Can you work these out from the model? Positions are in its coordinate system, mm. Face numbers are marked on the shaded views. A direction names the side the tool comes from. Give positions to 0.01 mm unless a question says otherwise; leave off trailing zeros. Order: outer loops, then holes, each group sorted by start corner. A loop starts at its lowest first (then second) coordinate and runs counter-clockwise, first axis right, second up. Notation, with made-up numbers: (44.5, 62.25) -> (62.5, 62.25) arc R31 ccw to (62.5, 92.25) -> close; hole circle Ø10 at (40.25, -30). An arc over 180 degrees is marked (long way). Answer as CSV lines item,"result".
```python
from build123d import *

# Parameters (mm, degrees)
SKETCH2_OUTSIDE_W                   = 55.422
SKETCH2_OUTSIDE_H                   = 55.422
CUT_EXTRUDE_PUSHER_SIDE_CROSS_DEPTH = 103.124
CUT_EXTRUDE_CROSS_2_DEPTH           = 3.048
SKETCH8_OUTSIDE_W                   = 55.422
SKETCH8_OUTSIDE_H                   = 55.422
CUT_EXTRUDE1_DEPTH                  = 3.54


with BuildPart() as part:
    # Sketch1 → Revolve: Main Body (revolve)
    with BuildSketch(Plane.XY):
        with BuildLine():
            Line((0, 0), (0, 14.605))
            Line((0, 14.605), (1.651, 14.605))
            Line((1.651, 14.605), (1.651, 11.7348))
            Line((1.651, 11.7348), (106.68, 11.7348))
            Line((106.68, 11.7348), (106.68, 9.5885))
            Line((106.68, 9.5885), (111.252, 9.5885))
            Line((111.252, 9.5885), (111.252, 8.89))
            Line((111.252, 8.89), (113.775706947, 1.318879159))
            ThreePointArc((113.775706947, 1.318879159), (113.787900268, 1.269334705), (113.792, 1.218476843))
            Line((113.792, 1.218476843), (113.792, 0))
            Line((113.792, 0), (0, 0))
        make_face()
    revolve(axis=Axis((-3.305576832, 0, 0), (1, 0, 0)))

    # Sketch2 outside → Cut-Extrude: Pusher Side Cross (cut)
    with BuildSketch(Plane(origin=(1.651, 0, 0), x_dir=(0, 0, -1), z_dir=(1, 0, 0))):
        Rectangle(SKETCH2_OUTSIDE_W, SKETCH2_OUTSIDE_H)
        Polygon((-0.6985, 11.303), (0.6985, 11.303), (0.6985, 0.6985), (11.303, 0.6985), (11.303, -0.6985), (0.6985, -0.6985), (0.6985, -11.303), (-0.6985, -11.303), (-0.6985, -0.6985), (-11.303, -0.6985), (-11.303, 0.6985), (-0.6985, 0.6985), align=None, mode=Mode.SUBTRACT)
    extrude(amount=CUT_EXTRUDE_PUSHER_SIDE_CROSS_DEPTH, mode=Mode.SUBTRACT)

    # Sketch3 → Cut-Extrude: Cross 2 (cut)
    with BuildSketch(Plane(origin=(106.68, 0, 0), x_dir=(0, 0, -1), z_dir=(1, 0, 0))):
        with BuildLine():
            Line((-11.713992863, 0.6985), (-9.563024103, 0.6985))
            ThreePointArc((-9.563024103, 0.6985), (-6.780093371, 6.780093371), (-0.6985, 9.563024103))
            Line((-0.6985, 9.563024103), (-0.6985, 11.713992863))
            ThreePointArc((-0.6985, 11.713992863), (-8.297756656, 8.297756656), (-11.713992863, 0.6985))
        make_face()
        with BuildLine():
            Line((0.6985, 11.713992863), (0.6985, 9.563024103))
            ThreePointArc((0.6985, 9.563024103), (6.780093371, 6.780093371), (9.563024103, 0.6985))
            Line((9.563024103, 0.6985), (11.713992863, 0.6985))
            ThreePointArc((11.713992863, 0.6985), (8.297756656, 8.297756656), (0.6985, 11.713992863))
        make_face()
        with BuildLine():
            ThreePointArc((9.563024103, -0.6985), (6.780093371, -6.780093371), (0.6985, -9.563024103))
            Line((0.6985, -9.563024103), (0.6985, -11.713992863))
            ThreePointArc((0.6985, -11.713992863), (8.297756656, -8.297756656), (11.713992863, -0.6985))
            Line((11.713992863, -0.6985), (9.563024103, -0.6985))
        make_face()
        with BuildLine():
            ThreePointArc((-0.6985, -9.563024103), (-6.780093371, -6.780093371), (-9.563024103, -0.6985))
            Line((-9.563024103, -0.6985), (-11.713992863, -0.6985))
            ThreePointArc((-11.713992863, -0.6985), (-8.297756656, -8.297756656), (-0.6985, -11.713992863))
            Line((-0.6985, -11.713992863), (-0.6985, -9.563024103))
        make_face()
        with BuildLine():
            Line((-9.563024103, 0.6985), (-7.58791788, 0.6985))
            Line((-7.58791788, 0.6985), (-0.6985, 0.6985))
            Line((-0.6985, 0.6985), (-0.6985, 7.58791788))
            Line((-0.6985, 7.58791788), (-0.6985, 9.563024103))
            ThreePointArc((-0.6985, 9.563024103), (-6.780093371, 6.780093371), (-9.563024103, 0.6985))
        make_face()
        with BuildLine():
            Line((0.6985, 9.563024103), (0.6985, 7.58791788))
            Line((0.6985, 7.58791788), (0.6985, 0.6985))
            Line((0.6985, 0.6985), (7.58791788, 0.6985))
            Line((7.58791788, 0.6985), (9.563024103, 0.6985))
            ThreePointArc((9.563024103, 0.6985), (6.780093371, 6.780093371), (0.6985, 9.563024103))
        make_face()
        with BuildLine():
            Line((0.6985, -7.58791788), (0.6985, -9.563024103))
            ThreePointArc((0.6985, -9.563024103), (6.780093371, -6.780093371), (9.563024103, -0.6985))
            Line((9.563024103, -0.6985), (7.58791788, -0.6985))
            Line((7.58791788, -0.6985), (0.6985, -0.6985))
            Line((0.6985, -0.6985), (0.6985, -7.58791788))
        make_face()
        with BuildLine():
            Line((-0.6985, -0.6985), (-7.58791788, -0.6985))
            Line((-7.58791788, -0.6985), (-9.563024103, -0.6985))
            ThreePointArc((-9.563024103, -0.6985), (-6.780093371, -6.780093371), (-0.6985, -9.563024103))
            Line((-0.6985, -9.563024103), (-0.6985, -7.58791788))
            Line((-0.6985, -7.58791788), (-0.6985, -0.6985))
        make_face()
        with BuildLine():
            Line((-0.6985, -7.58791788), (-0.6985, -9.563024103))
            ThreePointArc((-0.6985, -9.563024103), (0, -9.5885), (0.6985, -9.563024103))
            Line((0.6985, -9.563024103), (0.6985, -7.58791788))
            ThreePointArc((0.6985, -7.58791788), (0, -7.62), (-0.6985, -7.58791788))
        make_face()
        with BuildLine():
            Line((-0.6985, 9.563024103), (-0.6985, 7.58791788))
            ThreePointArc((-0.6985, 7.58791788), (0, 7.62), (0.6985, 7.58791788))
            Line((0.6985, 7.58791788), (0.6985, 9.563024103))
            ThreePointArc((0.6985, 9.563024103), (0, 9.5885), (-0.6985, 9.563024103))
        make_face()
        with BuildLine():
            Line((-0.6985, 11.713992863), (-0.6985, 9.563024103))
            ThreePointArc((-0.6985, 9.563024103), (0, 9.5885), (0.6985, 9.563024103))
            Line((0.6985, 9.563024103), (0.6985, 11.713992863))
            ThreePointArc((0.6985, 11.713992863), (0, 11.7348), (-0.6985, 11.713992863))
        make_face()
        with BuildLine():
            ThreePointArc((0.6985, -9.563024103), (0, -9.5885), (-0.6985, -9.563024103))
            Line((-0.6985, -9.563024103), (-0.6985, -11.713992863))
            ThreePointArc((-0.6985, -11.713992863), (0, -11.7348), (0.6985, -11.713992863))
            Line((0.6985, -11.713992863), (0.6985, -9.563024103))
        make_face()
        with BuildLine():
            Line((11.713992863, 0.6985), (9.563024103, 0.6985))
            ThreePointArc((9.563024103, 0.6985), (9.582128909, 0.349482214), (9.5885, 0))
            ThreePointArc((9.5885, 0), (9.582128909, -0.349482214), (9.563024103, -0.6985))
            Line((9.563024103, -0.6985), (11.713992863, -0.6985))
            ThreePointArc((11.713992863, -0.6985), (11.729597062, -0.349404918), (11.7348, 0))
            ThreePointArc((11.7348, 0), (11.729597062, 0.349404918), (11.713992863, 0.6985))
        make_face()
        with BuildLine():
            ThreePointArc((9.5885, 0), (9.582128909, 0.349482214), (9.563024103, 0.6985))
            Line((9.563024103, 0.6985), (7.58791788, 0.6985))
            ThreePointArc((7.58791788, 0.6985), (7.62, 0), (7.58791788, -0.6985))
            Line((7.58791788, -0.6985), (9.563024103, -0.6985))
            ThreePointArc((9.563024103, -0.6985), (9.582128909, -0.349482214), (9.5885, 0))
        make_face()
        with BuildLine():
            ThreePointArc((-7.58791788, -0.6985), (-7.62, 0), (-7.58791788, 0.6985))
            Line((-7.58791788, 0.6985), (-9.563024103, 0.6985))
            ThreePointArc((-9.563024103, 0.6985), (-9.5885, 0), (-9.563024103, -0.6985))
            Line((-9.563024103, -0.6985), (-7.58791788, -0.6985))
        make_face()
        with BuildLine():
            ThreePointArc((-9.563024103, -0.6985), (-9.5885, 0), (-9.563024103, 0.6985))
            Line((-9.563024103, 0.6985), (-11.713992863, 0.6985))
            ThreePointArc((-11.713992863, 0.6985), (-11.7348, 0), (-11.713992863, -0.6985))
            Line((-11.713992863, -0.6985), (-9.563024103, -0.6985))
        make_face()
    extrude(amount=CUT_EXTRUDE_CROSS_2_DEPTH, mode=Mode.SUBTRACT)

    # Sketch8 outside → Cut-Extrude1 (cut, through all)
    with BuildSketch(Plane(origin=(111.252, 0, 0), x_dir=(0, 0, -1), z_dir=(1, 0, 0))):
        Rectangle(SKETCH8_OUTSIDE_W, SKETCH8_OUTSIDE_H)
        with BuildLine():
            Line((-0.6985, -14.588287177), (0.6985, -14.588287177))
            Line((0.6985, -14.588287177), (0.6985, -1.016))
            ThreePointArc((0.6985, -1.016), (0.791493597, -0.791493597), (1.016, -0.6985))
            Line((1.016, -0.6985), (14.588287177, -0.6985))
            Line((14.588287177, -0.6985), (14.588287177, 0.6985))
            Line((14.588287177, 0.6985), (1.016, 0.6985))
            ThreePointArc((1.016, 0.6985), (0.791493597, 0.791493597), (0.6985, 1.016))
            Line((0.6985, 1.016), (0.6985, 14.588287177))
            Line((0.6985, 14.588287177), (-0.6985, 14.588287177))
            Line((-0.6985, 14.588287177), (-0.6985, 1.016))
            ThreePointArc((-0.6985, 1.016), (-0.791493597, 0.791493597), (-1.016, 0.6985))
            Line((-1.016, 0.6985), (-14.588287177, 0.6985))
            Line((-14.588287177, 0.6985), (-14.588287177, -0.6985))
            Line((-14.588287177, -0.6985), (-1.016, -0.6985))
            ThreePointArc((-1.016, -0.6985), (-0.791493597, -0.791493597), (-0.6985, -1.016))
            Line((-0.6985, -1.016), (-0.6985, -14.588287177))
        make_face(mode=Mode.SUBTRACT)
    extrude(amount=CUT_EXTRUDE1_DEPTH, mode=Mode.SUBTRACT)


solid = part.part
```
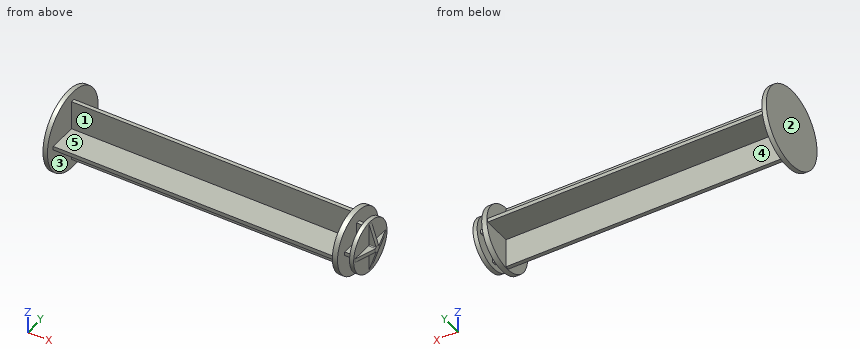
Item 1: For the marked faces 3, 4 and 5, which set-ups out of +Z, -Z, +X, -X, +Y, -Y let a thin tool reach every point of the face, with its end or its side?
Numbers:
face 3,"none"
face 4,"-Z, +Y"
face 5,"+Z, -Y"
Item 2: Imagine slicing it at A-A, the plane x = 26. Please give me the cut outline in (y, z), then the cut area to 3 significant figures.
Numbers:
outline,"(-11.3, -0.7) -> (-0.7, -0.7) -> (-0.7, -11.3) -> (0.7, -11.3) -> (0.7, -0.7) -> (11.3, -0.7) -> (11.3, 0.7) -> (0.7, 0.7) -> (0.7, 11.3) -> (-0.7, 11.3) -> (-0.7, 0.7) -> (-11.3, 0.7) -> close"
area,"61.2 mm²"
Item 3: We'd pull the mould along X, two halves only. Please class the marked faces 1 and 2: released by +X, released by -X, zero draft, split by the parting line, or undercut.
Numbers:
face 1,"undercut"
face 2,"released by -X"
Item 4: Please list where these lines run through material, in increasing order: line 1 along X through (y, z) = (1.5, -6.5) (3 decimals); line 2 along X through (y, z) = (-9, 5.25) (3 decimals); line 3 along X through (y, z) = (-8, 10).
Numbers:
line 1,"x = 0 to 1.651, 104.775 to 106.68, 109.728 to 111.252"
line 2,"x = 0 to 1.651, 104.775 to 106.68"
line 3,"x = 0 to 1.65"
Item 5: For pin 1 (2 mm diameter, centred on x = 113, z = -3.5, fed in from -Y); pin 2 (5 mm diameter, centred on x = 49, y = 11, fed in from +Z); pin 3 (1.5 mm diameter, centred on x = 69, y = -0.5, fed in from +Z), each with a flat end and sliding along its axis, tell me the tip position at first contact or that it passes through.
Numbers:
pin 1,"stops at y = -0.7"
pin 2,"stops at z = 0.7"
pin 3,"stops at z = 11.3"
Item 6: Imagine slicing it at B-B, the plane z = 12.75. Please give me the cut outline in (x, y), then the cut area to 3 significant figures.
Numbers:
outline,"(0, -7.12) -> (1.65, -7.12) -> (1.65, 7.12) -> (0, 7.12) -> close"
area,"23.5 mm²"
